Build history of the part. All positions in model axes, mm. A direction names the side the tool comes from. Round coordinates to 2 decimals unless told otherwise and drop trailing zeros. Write each loop counter-clockwise with the first axis right and the second up, starting at its lowest first coordinate (ties: lowest second). Pieces come first, ordered by that corner, then holes. Notation, with made-up numbers: M 48,68.5 L 78,68.5 A18 cw 78,74.5 Z; hole C -11.5,59.25 d3. An arc over 180 degrees is marked long. Use a Markdown table: item, result.
from build123d import *

# Parameters (mm, degrees)
SKETCH_1_W          = 20
SKETCH_1_H          = 20
SKETCH_1_W_2        = 16
SKETCH_1_H_2        = 16
EXTRUDE_1_DEPTH     = 970
SKETCH_2_R          = 2.2
SKETCH_2_R_2        = 5.5
CUT_EXTRUDE_1_DEPTH = 970
SKETCH_3_R          = 2.2
CUT_EXTRUDE_2_DEPTH = 970


with BuildPart() as part:
    # ｽｹｯﾁ1 → ﾎﾞｽ - 押し出し1 (new body)
    with BuildSketch(Plane.XY):
        Rectangle(SKETCH_1_W, SKETCH_1_H)
        Rectangle(SKETCH_1_W_2, SKETCH_1_H_2, mode=Mode.SUBTRACT)
    extrude(amount=EXTRUDE_1_DEPTH)

    # ｽｹｯﾁ2 → ｶｯﾄ - 押し出し1 (cut)
    with BuildSketch(Plane(origin=(10, 0, 0), x_dir=(0, 0, -1), z_dir=(1, 0, 0))):
        with Locations((-710, 0)):
            Circle(SKETCH_2_R)
        with Locations((-670, 0)):
            Circle(SKETCH_2_R)
        with Locations((-50, 0)):
            Circle(SKETCH_2_R)
        with Locations((-30, 0)):
            Circle(SKETCH_2_R_2)
    extrude(amount=-CUT_EXTRUDE_1_DEPTH, mode=Mode.SUBTRACT)

    # ｽｹｯﾁ3 → ｶｯﾄ - 押し出し2 (cut)
    with BuildSketch(Plane(origin=(0, 10, 0), x_dir=(1, 0, 0), z_dir=(0, 1, 0))):
        with Locations((0, -690)):
            Circle(SKETCH_3_R)
        with Locations((0, -660)):
            Circle(SKETCH_3_R)
        with Locations((0, -10)):
            Circle(SKETCH_3_R)
    extrude(amount=-CUT_EXTRUDE_2_DEPTH, mode=Mode.SUBTRACT)


solid = part.part
Q1. Cut at A-A on z = 281.5. Give the cut face in (x, y).
Response values:
| item | result |
|---|---|
| outline | M -10,-10 L 10,-10 L 10,10 L -10,10 Z; hole M -8,-8 L 8,-8 L 8,8 L -8,8 Z |
Q2. Which spindle directions (+Z, -Z, +X, -X, +Y, -Y) get a long thin tool onto all of the face, cutting with end or side? Do faces 5 (the flat face through (0, -10, 478)), 6 (the flat face through (0, 8, 478)). Say none if no direction does.
Response values:
| item | result |
|---|---|
| face 5 | +Z, -Z, +X, -X, -Y |
| face 6 | +Z, -Z |
Q3. Drill centre lines: L1, parallel to X at y = 6.5, z = 493.5; L2, parallel to X at y = 8.8, z = 10. Where is each one in solid material? Low to high.
Response values:
| item | result |
|---|---|
| L1 | x = -10 to -8, 8 to 10 |
| L2 | x = -10 to -2.2, 2.2 to 10 |
Q4. Two-plate mould, pull along X, no slides. Class faces 1 (the flat face through (-10, 0, 478)), 2 (the flat face through (10, 0, 478)), 3 (the flat face through (8, 0, 478)), 4 (the flat face through (-9, 0, 970)): +X half, -X half, draft (parallel to the pull), parting line (faces both ways), or undercut.
Response values:
| item | result |
|---|---|
| face 1 | -X half |
| face 2 | +X half |
| face 3 | undercut |
| face 4 | draft |
Q5. Drop flat-ended pins along their axis: P1, Ø9, axis at y = 0, z = 30, coming from the +X side; P2, Ø5.5, axis at y = 0, z = 670, coming from the +X side. Give the stop position or say it passes through.
Response values:
| item | result |
|---|---|
| P1 | passes through |
| P2 | stops at x = 10 |
